Geometry check sheet. Reference: the model listing, model coordinates, mm. Face numbers are marked on the shaded views. Coordinates: 2 decimals unless noted, no trailing zeros. Order: outer loops, then holes, each group sorted by start corner. A loop starts at its lowest first (then second) coordinate and runs counter-clockwise, first axis right, second up. Notation, with made-up numbers: (-37.5, 27.25) - (11.5, 27.25) arc R22 ccw to (11.5, 64.25) - close; hole circle Ø3 at (60, 73.25). An arc over 180 degrees is marked (long way). Put each result on its own line as item: value.
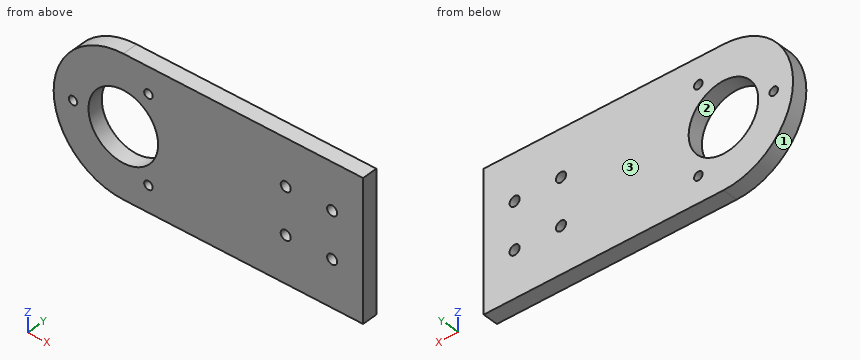
from build123d import *

# Parameters (mm, degrees)
BOSS_EXTRUDE1_DEPTH = 10
SKETCH2_R           = 2.75
SKETCH2_R_2         = 22.5
CUT_EXTRUDE1_DEPTH  = 11
SKETCH3_R           = 3.25
CUT_EXTRUDE2_DEPTH  = 11


with BuildPart() as part:
    # Sketch1 → Boss-Extrude1 (new body)
    with BuildSketch(Plane(origin=(0, 0, 0), x_dir=(1, 0, 0), z_dir=(0, 1, 0))):
        with BuildLine():
            Line((100, 45), (-55, 45))
            ThreePointArc((-55, 45), (-100, 0), (-55, -45))
            Line((-55, -45), (100, -45))
            Line((100, -45), (100, 45))
        make_face()
    extrude(amount=BOSS_EXTRUDE1_DEPTH)

    # Sketch2 → Cut-Extrude1 (cut, through all)
    with BuildSketch(Plane(origin=(0, 10, 0), x_dir=(1, 0, 0), z_dir=(0, 1, 0))):
        with Locations((-87.5, 0)):
            Circle(SKETCH2_R)
        with Locations((-38.75, 28.145825623)):
            Circle(SKETCH2_R)
        with Locations((-38.75, -28.145825623)):
            Circle(SKETCH2_R)
        with Locations((-55, 0)):
            Circle(SKETCH2_R_2)
    extrude(amount=-CUT_EXTRUDE1_DEPTH, mode=Mode.SUBTRACT)

    # Sketch3 → Cut-Extrude2 (cut, through all)
    with BuildSketch(Plane(origin=(0, 10, 0), x_dir=(1, 0, 0), z_dir=(0, 1, 0))):
        with Locations((80, 15)):
            Circle(SKETCH3_R)
        with Locations((50, 15)):
            Circle(SKETCH3_R)
        with Locations((50, -15)):
            Circle(SKETCH3_R)
        with Locations((80, -15)):
            Circle(SKETCH3_R)
    extrude(amount=-CUT_EXTRUDE2_DEPTH, mode=Mode.SUBTRACT)


solid = part.part
Q1. Section check D-D on x = -38.75. Record the boundary of the cut face in (y, z), then the cut area to 3 significant figures.
Answer block:
outline: (0, -45) - (10, -45) - (10, -30.9) - (0, -30.9) - close; (0, -25.4) - (10, -25.4) - (10, -15.56) - (0, -15.56) - close; (0, 15.56) - (10, 15.56) - (10, 25.4) - (0, 25.4) - close; (0, 30.9) - (10, 30.9) - (10, 45) - (0, 45) - close
area: 479 mm^2
Q2. Thickness scan on L1, parallel to Z at x = 50, y = 7.75; L2, parallel to Z at x = -55, y = 4.25; L3, parallel to X at y = 5.25, z = -15. Record the ranges inside material, lowest first. Write a range as [from, to].
Answer block:
L1: z = [-45, -18.25], [-11.75, 11.75], [18.25, 45]
L2: z = [-45, -22.5], [22.5, 45]
L3: x = [-97.43, -71.77], [-38.23, 46.75], [53.25, 76.75], [83.25, 100]
Q3. Section check A-A on x = 80. Record the boundary of the cut face in (y, z).
Answer block:
outline: (0, -45) - (10, -45) - (10, -18.25) - (0, -18.25) - close; (0, -11.75) - (10, -11.75) - (10, 11.75) - (0, 11.75) - close; (0, 18.25) - (10, 18.25) - (10, 45) - (0, 45) - close
Q4. Depth check by flat-ended pin: pin 1 Ø3.5 at (x, z) = (-87.5, 0) entering from -Y; pin 2 Ø2 at (y, z) = (2.5, -28.5) entering from -X. Enter the tip coordinate at first touch or a pass-through.
Answer block:
pin 1: passes through
pin 2: stops at x = -90.62
Q5. Draft check along Z on the marked faces 1, 2 and 3. Enter one of: pulls with the +Z half, pulls with the -Z half, needs draft (parallel to the pull), parting line crosses it, or undercut.
Answer block:
face 1: parting line crosses it
face 2: undercut
face 3: needs draft
Q6. Section check B-B on z = 0. Record the boundary of the cut face in (x, y), then the cut area to 4 significant figures.
Answer block:
outline: (-100, 0) - (-90.25, 0) - (-90.25, 10) - (-100, 10) - close; (-84.75, 0) - (-77.5, 0) - (-77.5, 10) - (-84.75, 10) - close; (-32.5, 0) - (100, 0) - (100, 10) - (-32.5, 10) - close
area: 1,495 mm^2
Q7. Section check C-C on y = 3.5. State how many separate pieces and enclosed holes the cut face has, then the cut area to 3 significant figures.
Answer block:
separate pieces: 1
enclosed holes: 8
area: 15,300 mm^2
